The drawing under review shows one solid part. Ordinate dimensions are in mm from its lowest x, y, z. A direction names the side the tool comes from. Give positions to 0.01 mm unless a question says otherwise; leave off trailing zeros. Order: outer loops, then holes, each group sorted by start corner. A loop starts at its lowest first (then second) coordinate and runs counter-clockwise, first axis right, second up. Notation, with made-up numbers: (-28, 33) -> (24, 33) arc R8 ccw to (24, 38) -> close; hole circle Ø3 at (16.25, 58). An arc over 180 degrees is marked (long way). Return JSON: item names as keys, results as strings. Group by question number.
1) Add section C-C (y = 12.4). Give the boundary of the cut face in (x, z), then the cut area to 3 significant figures.
2) To check wall thickness, follow line 1 along Y through (x, z) = (42, 1.35); line 2 along Y through (x, z) = (14, 0.9); line 3 along X through (y, z) = (27.5, 7). State the ranges of each line that lie inside material, in increasing order.
3) Add section B-B (x = 46). Give the boundary of the cut face in (y, z).
4) The part is to be moulded in two halves that separate along X. For the marked faces 1, 2 and 3, say which applies: released by +X, released by -X, zero draft, split by the parting line, or undercut.
5) Insertion check: P1, Ø5.5, axis at x = 14, y = 29.6, coming from the +Z side; P2, Ø2, axis at x = 19.5, y = 9.5, coming from the +Z side. Each pin has a flat end and moves straight along its axis. Give the tip position at first contact, or say it passes through.
6) Add section D-D (x = 14). Give the boundary of the cut face in (y, z).
7) Add section A-A (z = 9.25). Give the boundary of the cut face in (x, y), then the cut area to 3 significant figures.
8) For the marked faces 4 and 5, list the 3-axis set-ups (+Z, -Z, +X, -X, +Y, -Y) from which the entire face can be reached by the end or side of a thin tool; tool diameter is ignored.
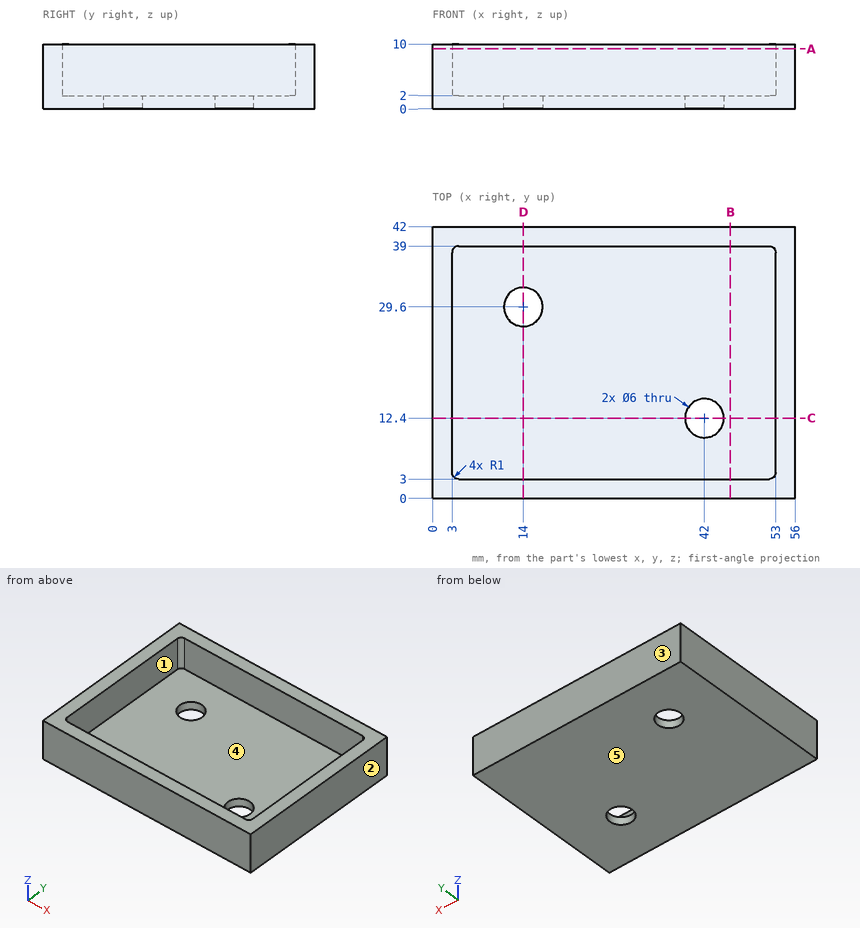
Evaluation:
{
 "1": {"outline": "(0, 0) -> (39, 0) -> (39, 2) -> (3, 2) -> (3, 10) -> (0, 10) -> close; (45, 0) -> (56, 0) -> (56, 10) -> (53, 10) -> (53, 2) -> (45, 2) -> close", "area": "148 mm^2"},
 "2": {"line 1": "0 to 9.4, 15.4 to 42", "line 2": "0 to 26.6, 32.6 to 42", "line 3": "0 to 3, 53 to 56"},
 "3": {"outline": "(0, 0) -> (42, 0) -> (42, 10) -> (39, 10) -> (39, 2) -> (3, 2) -> (3, 10) -> (0, 10) -> close"},
 "4": {"face 1": "undercut", "face 2": "released by +X", "face 3": "zero draft"},
 "5": {"P1": "through", "P2": "z = 2"},
 "6": {"outline": "(0, 0) -> (26.6, 0) -> (26.6, 2) -> (3, 2) -> (3, 10) -> (0, 10) -> close; (32.6, 0) -> (42, 0) -> (42, 10) -> (39, 10) -> (39, 2) -> (32.6, 2) -> close"},
 "7": {"outline": "(0, 0) -> (56, 0) -> (56, 42) -> (0, 42) -> close; hole (3, 4) arc R1 ccw to (4, 3) -> (52, 3) arc R1 ccw to (53, 4) -> (53, 38) arc R1 ccw to (52, 39) -> (4, 39) arc R1 ccw to (3, 38) -> close", "area": "553 mm^2"},
 "8": {"face 4": "+Z", "face 5": "-Z, +X, -X, +Y, -Y"}
}
